Design review of the part built by this model. Coordinates are the model's own, in mm. Face numbers are marked on the shaded views. A direction names the side the tool comes from. Coordinates: 2 decimals unless noted, no trailing zeros. Loops run counter-clockwise (first coordinate to the right, second up) from the corner with the lowest first, then second, coordinate; pieces in that order, holes last. Notation, with made-up numbers: M 71.5,69.5 L 130.5,69.5 A19 cw 130.5,103.5 Z; hole C 66.25,51.25 d2. An arc over 180 degrees is marked long. Write item = value, one per line. Start each with the question number.
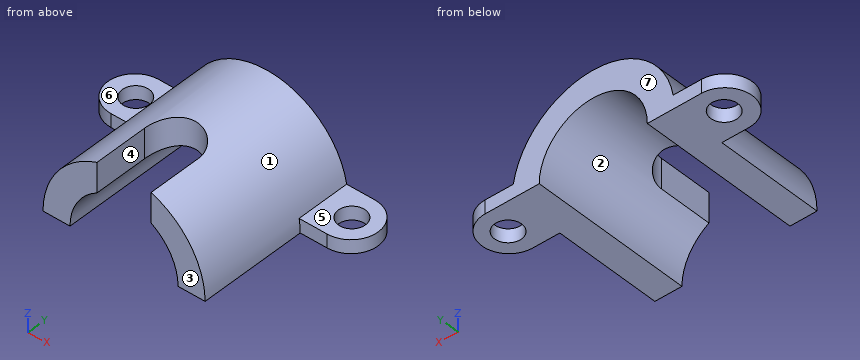
```python
from build123d import *

# Parameters (mm, degrees)
F0_R      = 30
F1_DEPTH  = 60
F3_DEPTH  = 60
F4_R      = 5
F5_DEPTH  = 5
F7_DEPTH  = 60
F10_W     = 20
F10_H     = 40
F11_DEPTH = 25


with BuildPart() as f1:
    # F0 (on Front) → F1 (new body)
    with BuildSketch(Plane.XZ):
        Circle(F0_R)
    extrude(amount=F1_DEPTH)

    # F2 (on face) → F3 (cut, through all)
    with BuildSketch(Plane.XZ.offset(60)):
        with BuildLine():
            Line((30, 0), (-30, 0))
            ThreePointArc((-30, 0), (0, -30), (30, 0))
        make_face()
    extrude(amount=-F3_DEPTH, mode=Mode.SUBTRACT)

    # F4 (on Top) → F5 (join)
    with BuildSketch(Plane.XY):
        with BuildLine():
            Line((40, 0), (-40, 0))
            ThreePointArc((-40, 0), (-50, -10), (-40, -20))
            Line((-40, -20), (40, -20))
            ThreePointArc((40, -20), (50, -10), (40, 0))
        make_face()
        with Locations((-39.6707831735, -10)):
            Circle(F4_R, mode=Mode.SUBTRACT)
        with Locations((40.3292197076, -10)):
            Circle(F4_R, mode=Mode.SUBTRACT)
    extrude(amount=F5_DEPTH)

    # F6 (on face) → F7 (cut, through all)
    with BuildSketch(Plane.XZ.offset(60)):
        with BuildLine():
            Line((-20, 0), (20, 0))
            ThreePointArc((20, 0), (0, 20), (-20, 0))
        make_face()
    extrude(amount=-F7_DEPTH, mode=Mode.SUBTRACT)

    # F10 (on plane+point) → F11 (cut)
    with BuildSketch(Plane.XY.offset(30)):
        with BuildLine():
            Line((-10, -40), (10, -40))
            ThreePointArc((10, -40), (0, -30), (-10, -40))
        make_face()
        with Locations((0, -60)):
            Rectangle(F10_W, F10_H)
    extrude(amount=-F11_DEPTH, mode=Mode.SUBTRACT)


solid = f1.part
```
(1) Take a section at B-B (y = -10). State the section outline as (x, z) points, plus the area to 3 significant figures.
(2) Tool access review of the marked faces 4, 5, 6 and 7: name each direction out of +Z, -Z, +X, -X, +Y, -Y from which nothing blocks a thin tool from reaching the whole face with its end or side.
(3) Insertion check: pin 1 (1.5 mm diameter, centred on y = -46, z = 10.5, fed in from +X); pin 2 (4 mm diameter, centred on x = -14, y = -35, fed in from +Z); pin 3 (1.5 mm diameter, centred on x = 24, z = 13, fed in from +Y); pin 4 (1.5 mm diameter, centred on x = -33, z = 1.5, fed in from -Y). Each pin has a flat end and moves straight along its axis. Give the tip position at first contact, or say it passes through.
(4) To check wall thickness, follow L1, parallel to X at y = -7, z = 4.5; L2, parallel to Z at x = -37, y = -19.5; L3, parallel to X at y = -45, z = 23. State the ranges of each line that lie inside material, in increasing order.
(5) Mouldability with a two-part tool opening along X and no side actions: class the marked faces 1, 2 and 3 as +X half, -X half, draft (parallel to the pull), parting line (faces both ways), or undercut.
(6) Take a section at D-D (x = 33). State the section outline as (y, z) points, plus the area to 3 significant figures.
(7) Take a section at A-A (y = -42.5). State the section outline as (x, z) points.
(8) Take a section at C-C (z = 6). State the section outline as (x, y) points.
Results list:
q1.outline = M -50,0 L -44.67,0 L -44.67,5 L -50,5 Z; M -34.67,0 L -20,0 A20 cw 20,0 L 35.33,0 L 35.33,5 L 29.58,5 A30 ccw -29.58,5 L -34.67,5 Z; M 45.33,0 L 50,0 L 50,5 L 45.33,5 Z
q1.area = 887 mm^2
q2.face_4 = +Z, -Z, -Y
q2.face_5 = +Z, +X, +Y, -Y
q2.face_6 = +Z, -X, +Y, -Y
q2.face_7 = +Z, -Z, +X, -X, +Y
q3.pin_1 = 28.37
q3.pin_2 = 27.5
q3.pin_3 = 0
q3.pin_4 = -20
q4.L1 = -49.54 to -43.67, -35.67 to -19.49, 19.49 to 36.33, 44.33 to 49.54
q4.L2 = 0 to 5
q4.L3 = -19.26 to -10, 10 to 19.26
q5.face_1 = parting line
q5.face_2 = undercut
q5.face_3 = draft
q6.outline = M -20,0 L 0,0 L 0,5 L -20,5 Z
q6.area = 100 mm^2
q7.outline = M -30,0 L -20,0 A20 cw -10,17.32 L -10,28.28 A30 ccw Z; M 10,17.32 A20 cw 20,0 L 30,0 A30 ccw 10,28.28 Z
q8.outline = M -29.39,-60 L -19.08,-60 L -19.08,0 L -29.39,0 Z; M 19.08,-60 L 29.39,-60 L 29.39,0 L 19.08,0 Z
